Model file for the job. Use its own axes, mm. Give positions to 0.01 mm unless a question says otherwise; leave off trailing zeros. Loops run counter-clockwise (first coordinate to the right, second up) from the corner with the lowest first, then second, coordinate; pieces in that order, holes last. Notation, with made-up numbers: M -11.75,-10.5 L 28.25,-10.5 A22 cw 28.25,27.5 Z; hole C 53,89 d6. An arc over 180 degrees is marked long. Answer in a Markdown table with one row per item.
```python
from build123d import *

# Parameters (mm, degrees)
ESQUISSE1_W        = 6
ESQUISSE1_H        = 25
ESQUISSE1_R        = 1.55
BOSS_EXTRU_1_DEPTH = 6.35
CONG_1_R           = 2


with BuildPart() as part:
    # Esquisse1 → Boss.-Extru.1 (new body)
    with BuildSketch(Plane.XY):
        Rectangle(ESQUISSE1_W, ESQUISSE1_H)
        with Locations(Location((0, -9.837865065, 0), (0, 0, 180))):
            Circle(ESQUISSE1_R, mode=Mode.SUBTRACT)
        Circle(ESQUISSE1_R, mode=Mode.SUBTRACT)
        with Locations((0, 5)):
            Circle(ESQUISSE1_R, mode=Mode.SUBTRACT)
    extrude(amount=BOSS_EXTRU_1_DEPTH)

    # Congé1
    cong_1_edges = [part.edges().sort_by_distance(p)[0] for p in [
        (3, -12.5, 3.175),
        (-3, -12.5, 3.175),
        (-3, 12.5, 3.175),
        (3, 12.5, 3.175),
    ]]
    fillet(cong_1_edges, radius=CONG_1_R)


solid = part.part
```
(1) Saw through at D-D, the plane y = 0.5. Give the cut face in (x, z), and give its area (3 significant figures).
Established:
| item | result |
|---|---|
| outline | M -3,0 L -1.47,0 L -1.47,6.35 L -3,6.35 Z; M 1.47,0 L 3,0 L 3,6.35 L 1.47,6.35 Z |
| area | 19.5 mm2 |
(2) Flat gauge pin, fed straight in: P1, Ø2.5, axis at x = 0, y = 5, coming from the -Z side. Where does the tip first touch, or does it go through?
Established:
| item | result |
|---|---|
| P1 | passes through |
(3) Wall check: L1, parallel to Y at x = 0, z = 3.5; L2, parallel to Y at x = -0.75, z = 3.5; L3, parallel to X at y = -9.5, z = 4.5. Give the ranges that are in metal, low to high.
Established:
| item | result |
|---|---|
| L1 | y = -12.5 to -11.39, -8.29 to -1.55, 1.55 to 3.45, 6.55 to 12.5 |
| L2 | y = -12.5 to -11.19, -8.48 to -1.36, 1.36 to 3.64, 6.36 to 12.5 |
| L3 | x = -3 to -1.51, 1.51 to 3 |
(4) Saw through at C-C, the plane z = 2.5. Give the cut face in (x, y), and give its area (3 significant figures).
Established:
| item | result |
|---|---|
| outline | M -3,-10.5 A2 ccw -1,-12.5 L 1,-12.5 A2 ccw 3,-10.5 L 3,10.5 A2 ccw 1,12.5 L -1,12.5 A2 ccw -3,10.5 Z; hole C 0,-9.84 d3.1; hole C 0,0 d3.1; hole C 0,5 d3.1 |
| area | 124 mm2 |
(5) Saw through at A-A, the plane y = 5. Give the cut face in (x, z).
Established:
| item | result |
|---|---|
| outline | M -3,0 L -1.55,0 L -1.55,6.35 L -3,6.35 Z; M 1.55,0 L 3,0 L 3,6.35 L 1.55,6.35 Z |
(6) Saw through at B-B, the plane x = 0. Give the cut face in (y, z), and give its area (3 significant figures).
Established:
| item | result |
|---|---|
| outline | M -12.5,0 L -11.39,0 L -11.39,6.35 L -12.5,6.35 Z; M -8.29,0 L -1.55,0 L -1.55,6.35 L -8.29,6.35 Z; M 1.55,0 L 3.45,0 L 3.45,6.35 L 1.55,6.35 Z; M 6.55,0 L 12.5,0 L 12.5,6.35 L 6.55,6.35 Z |
| area | 99.7 mm2 |
(7) Mould opens along X. For faces 1 (the cylindrical face through (-2.43, 11.9, 3.22)), 2 (the flat face through (0, 12.5, 3)), 3 (the cylindrical face through (0.715, -1.375, 3.131)) say: pulls with the +X half, pulls with the -X half, needs draft (parallel to the pull), parting line crosses it, or undercut.
Established:
| item | result |
|---|---|
| face 1 | pulls with the -X half |
| face 2 | needs draft |
| face 3 | undercut |
